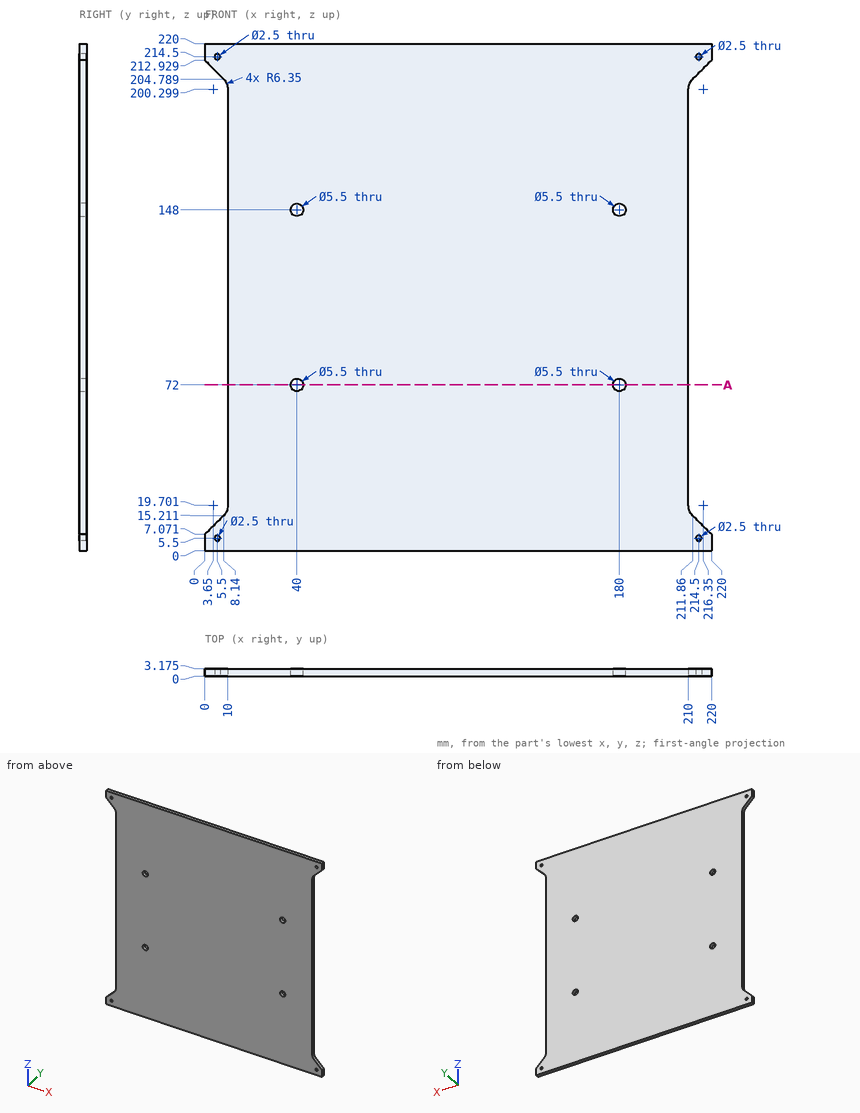
Here's the drawing with two shaded views (mm, measured from the low corner). I have some questions. Round coordinates to 2 decimals unless told otherwise and drop trailing zeros.
(1) If I drill on probe 1 along X at (y, z) = (1.85, 72); probe 2 along X at (y, z) = (1.65, 214.5); probe 3 along Z at (x, y) = (5.5, 1.8), over which ranges is the centre line in solid material (lowest first)?
Findings below:
probe 1: x = 10 to 37.25, 42.75 to 177.25, 182.75 to 210
probe 2: x = 0 to 4.25, 6.75 to 213.25, 215.75 to 220
probe 3: z = 0 to 4.25, 6.75 to 12.57, 207.43 to 213.25, 215.75 to 220
(2) Suppose I cut it at A-A on z = 72. State how many separate pieces and enclosed holes the cut face has, and give its area (3 significant figures).
Findings below:
separate pieces: 3
enclosed holes: 0
area: 600 mm2
(3) For pin 1 (9 mm diameter, centred on x = 180, z = 148, fed in from +Y) (3 decimals), with a flat end and sliding along its axis, tell me the tip position at first contact or that it passes through.
Findings below:
pin 1: stops at y = 3.175
